Design review of the part built by this model. Coordinates are the model's own, in mm. Face numbers are marked on the shaded views. A direction names the side the tool comes from. Round coordinates to 2 decimals unless told otherwise and drop trailing zeros. Write each loop counter-clockwise with the first axis right and the second up, starting at its lowest first coordinate (ties: lowest second). Pieces come first, ordered by that corner, then holes. Notation, with made-up numbers: (64, 0) -> (98, 0) arc R27 cw to (98, 33) -> close; hole circle Ø7 at (-10, 29.5). An arc over 180 degrees is marked (long way). Write item = value, one per line. Start each with the question number.
Item 1: To check wall thickness, follow L1, parallel to Z at x = -17, y = 37; L2, parallel to X at y = -9.5, z = 28; L3, parallel to Y at x = -3.5, z = 21. State the ranges of each line that lie inside material, in increasing order.
Item 2: Add section D-D, the plane y = -2. State the section outline as (x, z) points.
Item 3: Mouldability with a two-part tool opening along Z and no side actions: class the marked faces 3, 4 and 5 as released by +Z, released by -Z, zero draft, split by the parting line, or undercut.
Item 4: For pin 1 Ø3 at (x, y) = (18, -42.5) entering from -Z; pin 2 Ø5 at (x, z) = (-5.5, 9.5) entering from -Y; pin 3 Ø12 at (x, y) = (-1, -25) entering from -Z; pin 4 Ø1.5 at (x, z) = (6.5, 17) entering from +Y, all flat-tipped, find the tip position at first contact; note any pin that passes through.
Item 5: Machinability: for the marked faces 1 and 2, which of the approach directions +Z, -Z, +X, -X, +Y, -Y give a long, thin tool a straight path to every point of the face, cutting with its end or side? Answer none if there is none.
Item 6: Add section A-A, the plane z = 9. State the section outline as (x, y) points.
Item 7: Add section C-C, the plane z = 17. State the section outline as (x, y) points.
Item 8: Add section B-B, the plane y = 36.5. State the section outline as (x, z) points, then the cut area to 3 significant figures.
from build123d import *

# Parameters (mm, degrees)
F0_W           = 41
F0_H           = 90
F1_DEPTH       = 34
F2_W           = 35
F2_H           = 29
F3_DEPTH       = 86
F4_W           = 7
F4_H           = 6
F4_R           = 1.55
F4_R_2         = 4
F5_DEPTH       = 4
F6_W           = 5
F6_H           = 2.5
F6_W_2         = 3
F6_H_2         = 5
F7_DEPTH       = 2.5
F8_W           = 5
F8_H           = 27
F9_DEPTH       = 4
F10_T4_DEPTH   = 29
F10_T10_DEPTH  = 29
F10_T16_DEPTH  = 29
F10_T23_DEPTH  = 29
F10_T29_DEPTH  = 29
F10_T35_DEPTH  = 29
F10_T41_DEPTH  = 29
F10_T47_DEPTH  = 29
F10_T54_DEPTH  = 29
F10_T60_DEPTH  = 29
F10_T66_DEPTH  = 35
F10_T72_DEPTH  = 35
F10_T78_DEPTH  = 35
F10_T85_DEPTH  = 35
F10_T91_DEPTH  = 35
F10_T97_DEPTH  = 35
F10_T103_DEPTH = 35
F10_T109_DEPTH = 35
F10_T116_DEPTH = 35
F10_T122_DEPTH = 35


# Not quite as in the source:
# - a fillet or chamfer that OpenCascade refuses, or shapes differently, is made with other operations: its cross-section is extruded or revolved along the edge and cut away or added


with BuildPart() as f1:
    # F0 (on Top) → F1 (new body)
    with BuildSketch(Plane.XY):
        with Locations((-1.7023412511, 4.193077401)):
            Rectangle(F0_W, F0_H)
    extrude(amount=F1_DEPTH)

    # F2 (on face) → F3 (cut)
    with BuildSketch(Plane.XZ.offset(40.806922599)):
        with Locations((-1.7023412511, 17)):
            Rectangle(F2_W, F2_H)
    extrude(amount=-F3_DEPTH, mode=Mode.SUBTRACT)

    # F4 (on face) → F5 (cut, through all)
    with BuildSketch(Plane(origin=(0, 49.193077401, 0), x_dir=(-1, 0, 0), z_dir=(0, 1, 0))):
        with Locations((-11.2976587489, 7)):
            Rectangle(F4_W, F4_H)
        with Locations((-7.7976587489, 17)):
            Circle(F4_R)
        with Locations((1.7023412511, 25)):
            Circle(F4_R)
        with Locations((1.7023412511, 17)):
            Circle(F4_R_2)
        with Locations((1.7023412511, 9)):
            Circle(F4_R)
        with Locations((11.2023412511, 17)):
            Circle(F4_R)
        with Locations((14.7023412511, 27)):
            Rectangle(F4_W, F4_H)
    extrude(amount=-F5_DEPTH, mode=Mode.SUBTRACT)

    # F6 (on face) → F7 (join)
    with BuildSketch(Plane.XZ.offset(40.806922599)):
        with Locations((-1.7023412511, 32.75)):
            Rectangle(F6_W, F6_H)
        with Locations((-20.7023412511, 17)):
            Rectangle(F6_W_2, F6_H_2)
        with Locations((17.2976587489, 17)):
            Rectangle(F6_W_2, F6_H_2)
        with Locations((-1.7023412511, 1.25)):
            Rectangle(F6_W, F6_H)
    extrude(amount=F7_DEPTH)

    # F8 (on face) → F9 (join)
    with BuildSketch(Plane(origin=(0, 0, 0), x_dir=(1, 0, 0), z_dir=(0, 0, -1))):
        with Locations((-19.7023412511, -9.693077401)):
            Rectangle(F8_W, F8_H)
        with Locations((16.2976587489, -9.693077401)):
            Rectangle(F8_W, F8_H)
    extrude(amount=F9_DEPTH)

    # F10: chamfer of 3 on 4 edges, made by hand


with BuildPart() as f10_tool2:
    # F10_s3 → F10_t4 (new body)
    with BuildSketch(Plane.XY.offset(31.5)):
        Polygon((-16.2023412511, 45.193077401), (-19.2023412511, 42.193077401), (-19.2023412511, 45.193077401), align=None)
    extrude(amount=-F10_T4_DEPTH)

    split(bisect_by=Plane.YZ.offset(-18.2023412511), keep=Keep.TOP)

    split(bisect_by=Plane.XY.offset(30), keep=Keep.TOP)


with BuildPart() as f1_1:
    add(f1.part)

    # F10_t1: union F10_tool2
    add(f10_tool2.part)


with BuildPart() as f10_tool8:
    # F10_s9 → F10_t10 (new body)
    with BuildSketch(Plane.XY.offset(31.5)):
        Polygon((-16.2023412511, 45.193077401), (-19.2023412511, 42.193077401), (-19.2023412511, 45.193077401), align=None)
    extrude(amount=-F10_T10_DEPTH)

    split(bisect_by=Plane.YZ.offset(-18.2023412511), keep=Keep.BOTTOM)

    split(bisect_by=Plane.XY.offset(30), keep=Keep.TOP)


with BuildPart() as f1_2:
    add(f1_1.part)

    # F10_t7: union F10_tool8
    add(f10_tool8.part)


with BuildPart() as f10_tool14:
    # F10_s15 → F10_t16 (new body)
    with BuildSketch(Plane.XY.offset(31.5)):
        Polygon((-16.2023412511, 45.193077401), (-19.2023412511, 42.193077401), (-19.2023412511, 45.193077401), align=None)
    extrude(amount=-F10_T16_DEPTH)

    split(bisect_by=Plane.YZ.offset(-18.2023412511), keep=Keep.BOTTOM)

    split(bisect_by=Plane.XY.offset(24), keep=Keep.TOP)

    split(bisect_by=Plane.XY.offset(30), keep=Keep.BOTTOM)


with BuildPart() as f1_3:
    add(f1_2.part)

    # F10_t13: union F10_tool14
    add(f10_tool14.part)


with BuildPart() as f10_tool21:
    # F10_s22 → F10_t23 (new body)
    with BuildSketch(Plane.XY.offset(31.5)):
        Polygon((-16.2023412511, 45.193077401), (-19.2023412511, 42.193077401), (-19.2023412511, 45.193077401), align=None)
    extrude(amount=-F10_T23_DEPTH)

    split(bisect_by=Plane.YZ.offset(-18.2023412511), keep=Keep.TOP)

    split(bisect_by=Plane.XY.offset(24), keep=Keep.BOTTOM)


with BuildPart() as f1_4:
    add(f1_3.part)

    # F10_t20: union F10_tool21
    add(f10_tool21.part)


with BuildPart() as f10_tool27:
    # F10_s28 → F10_t29 (new body)
    with BuildSketch(Plane.XY.offset(31.5)):
        Polygon((-16.2023412511, 45.193077401), (-19.2023412511, 42.193077401), (-19.2023412511, 45.193077401), align=None)
    extrude(amount=-F10_T29_DEPTH)

    split(bisect_by=Plane.YZ.offset(-18.2023412511), keep=Keep.BOTTOM)

    split(bisect_by=Plane.XY.offset(24), keep=Keep.BOTTOM)


with BuildPart() as f1_5:
    add(f1_4.part)

    # F10_t26: union F10_tool27
    add(f10_tool27.part)


with BuildPart() as f10_tool33:
    # F10_s34 → F10_t35 (new body)
    with BuildSketch(Plane.XY.offset(2.5)):
        Polygon((12.7976587489, 45.193077401), (15.7976587489, 42.193077401), (15.7976587489, 45.193077401), align=None)
    extrude(amount=F10_T35_DEPTH)

    split(bisect_by=Plane.XY.offset(4), keep=Keep.BOTTOM)

    split(bisect_by=Plane.YZ.offset(14.7976587489), keep=Keep.BOTTOM)


with BuildPart() as f1_6:
    add(f1_5.part)

    # F10_t32: union F10_tool33
    add(f10_tool33.part)


with BuildPart() as f10_tool39:
    # F10_s40 → F10_t41 (new body)
    with BuildSketch(Plane.XY.offset(2.5)):
        Polygon((12.7976587489, 45.193077401), (15.7976587489, 42.193077401), (15.7976587489, 45.193077401), align=None)
    extrude(amount=F10_T41_DEPTH)

    split(bisect_by=Plane.XY.offset(4), keep=Keep.BOTTOM)

    split(bisect_by=Plane.YZ.offset(14.7976587489), keep=Keep.TOP)


with BuildPart() as f1_7:
    add(f1_6.part)

    # F10_t38: union F10_tool39
    add(f10_tool39.part)


with BuildPart() as f10_tool45:
    # F10_s46 → F10_t47 (new body)
    with BuildSketch(Plane.XY.offset(2.5)):
        Polygon((12.7976587489, 45.193077401), (15.7976587489, 42.193077401), (15.7976587489, 45.193077401), align=None)
    extrude(amount=F10_T47_DEPTH)

    split(bisect_by=Plane.XY.offset(4), keep=Keep.TOP)

    split(bisect_by=Plane.YZ.offset(14.7976587489), keep=Keep.TOP)

    split(bisect_by=Plane.XY.offset(10), keep=Keep.BOTTOM)


with BuildPart() as f1_8:
    add(f1_7.part)

    # F10_t44: union F10_tool45
    add(f10_tool45.part)


with BuildPart() as f10_tool52:
    # F10_s53 → F10_t54 (new body)
    with BuildSketch(Plane.XY.offset(2.5)):
        Polygon((12.7976587489, 45.193077401), (15.7976587489, 42.193077401), (15.7976587489, 45.193077401), align=None)
    extrude(amount=F10_T54_DEPTH)

    split(bisect_by=Plane.YZ.offset(14.7976587489), keep=Keep.BOTTOM)

    split(bisect_by=Plane.XY.offset(10), keep=Keep.TOP)


with BuildPart() as f1_9:
    add(f1_8.part)

    # F10_t51: union F10_tool52
    add(f10_tool52.part)


with BuildPart() as f10_tool58:
    # F10_s59 → F10_t60 (new body)
    with BuildSketch(Plane.XY.offset(2.5)):
        Polygon((12.7976587489, 45.193077401), (15.7976587489, 42.193077401), (15.7976587489, 45.193077401), align=None)
    extrude(amount=F10_T60_DEPTH)

    split(bisect_by=Plane.YZ.offset(14.7976587489), keep=Keep.TOP)

    split(bisect_by=Plane.XY.offset(10), keep=Keep.TOP)


with BuildPart() as f1_10:
    add(f1_9.part)

    # F10_t57: union F10_tool58
    add(f10_tool58.part)


with BuildPart() as f10_tool64:
    # F10_s65 → F10_t66 (new body)
    with BuildSketch(Plane.YZ.offset(15.7976587489)):
        Polygon((45.193077401, 28.5), (42.193077401, 31.5), (45.193077401, 31.5), align=None)
    extrude(amount=-F10_T66_DEPTH)

    split(bisect_by=Plane.YZ.offset(-11.2023412511), keep=Keep.TOP)

    split(bisect_by=Plane.XY.offset(30), keep=Keep.BOTTOM)


with BuildPart() as f1_11:
    add(f1_10.part)

    # F10_t63: union F10_tool64
    add(f10_tool64.part)


with BuildPart() as f10_tool70:
    # F10_s71 → F10_t72 (new body)
    with BuildSketch(Plane.YZ.offset(15.7976587489)):
        Polygon((45.193077401, 28.5), (42.193077401, 31.5), (45.193077401, 31.5), align=None)
    extrude(amount=-F10_T72_DEPTH)

    split(bisect_by=Plane.YZ.offset(-11.2023412511), keep=Keep.TOP)

    split(bisect_by=Plane.XY.offset(30), keep=Keep.TOP)


with BuildPart() as f1_12:
    add(f1_11.part)

    # F10_t69: union F10_tool70
    add(f10_tool70.part)


with BuildPart() as f10_tool76:
    # F10_s77 → F10_t78 (new body)
    with BuildSketch(Plane.YZ.offset(15.7976587489)):
        Polygon((45.193077401, 28.5), (42.193077401, 31.5), (45.193077401, 31.5), align=None)
    extrude(amount=-F10_T78_DEPTH)

    split(bisect_by=Plane.YZ.offset(-18.2023412511), keep=Keep.TOP)

    split(bisect_by=Plane.YZ.offset(-11.2023412511), keep=Keep.BOTTOM)

    split(bisect_by=Plane.XY.offset(30), keep=Keep.TOP)


with BuildPart() as f1_13:
    add(f1_12.part)

    # F10_t75: union F10_tool76
    add(f10_tool76.part)


with BuildPart() as f10_tool83:
    # F10_s84 → F10_t85 (new body)
    with BuildSketch(Plane.YZ.offset(15.7976587489)):
        Polygon((45.193077401, 28.5), (42.193077401, 31.5), (45.193077401, 31.5), align=None)
    extrude(amount=-F10_T85_DEPTH)

    split(bisect_by=Plane.YZ.offset(-18.2023412511), keep=Keep.BOTTOM)

    split(bisect_by=Plane.XY.offset(30), keep=Keep.BOTTOM)


with BuildPart() as f1_14:
    add(f1_13.part)

    # F10_t82: union F10_tool83
    add(f10_tool83.part)


with BuildPart() as f10_tool89:
    # F10_s90 → F10_t91 (new body)
    with BuildSketch(Plane.YZ.offset(15.7976587489)):
        Polygon((45.193077401, 28.5), (42.193077401, 31.5), (45.193077401, 31.5), align=None)
    extrude(amount=-F10_T91_DEPTH)

    split(bisect_by=Plane.YZ.offset(-18.2023412511), keep=Keep.BOTTOM)

    split(bisect_by=Plane.XY.offset(30), keep=Keep.TOP)


with BuildPart() as f1_15:
    add(f1_14.part)

    # F10_t88: union F10_tool89
    add(f10_tool89.part)


with BuildPart() as f10_tool95:
    # F10_s96 → F10_t97 (new body)
    with BuildSketch(Plane.YZ.offset(-19.2023412511)):
        Polygon((45.193077401, 5.5), (42.193077401, 2.5), (45.193077401, 2.5), align=None)
    extrude(amount=F10_T97_DEPTH)

    split(bisect_by=Plane.YZ.offset(7.7976587489), keep=Keep.BOTTOM)

    split(bisect_by=Plane.XY.offset(4), keep=Keep.TOP)


with BuildPart() as f1_16:
    add(f1_15.part)

    # F10_t94: union F10_tool95
    add(f10_tool95.part)


with BuildPart() as f10_tool101:
    # F10_s102 → F10_t103 (new body)
    with BuildSketch(Plane.YZ.offset(-19.2023412511)):
        Polygon((45.193077401, 5.5), (42.193077401, 2.5), (45.193077401, 2.5), align=None)
    extrude(amount=F10_T103_DEPTH)

    split(bisect_by=Plane.YZ.offset(7.7976587489), keep=Keep.BOTTOM)

    split(bisect_by=Plane.XY.offset(4), keep=Keep.BOTTOM)


with BuildPart() as f1_17:
    add(f1_16.part)

    # F10_t100: union F10_tool101
    add(f10_tool101.part)


with BuildPart() as f10_tool107:
    # F10_s108 → F10_t109 (new body)
    with BuildSketch(Plane.YZ.offset(-19.2023412511)):
        Polygon((45.193077401, 5.5), (42.193077401, 2.5), (45.193077401, 2.5), align=None)
    extrude(amount=F10_T109_DEPTH)

    split(bisect_by=Plane.YZ.offset(7.7976587489), keep=Keep.TOP)

    split(bisect_by=Plane.XY.offset(4), keep=Keep.BOTTOM)

    split(bisect_by=Plane.YZ.offset(14.7976587489), keep=Keep.BOTTOM)


with BuildPart() as f1_18:
    add(f1_17.part)

    # F10_t106: union F10_tool107
    add(f10_tool107.part)


with BuildPart() as f10_tool114:
    # F10_s115 → F10_t116 (new body)
    with BuildSketch(Plane.YZ.offset(-19.2023412511)):
        Polygon((45.193077401, 5.5), (42.193077401, 2.5), (45.193077401, 2.5), align=None)
    extrude(amount=F10_T116_DEPTH)

    split(bisect_by=Plane.XY.offset(4), keep=Keep.TOP)

    split(bisect_by=Plane.YZ.offset(14.7976587489), keep=Keep.TOP)


with BuildPart() as f1_19:
    add(f1_18.part)

    # F10_t113: union F10_tool114
    add(f10_tool114.part)


with BuildPart() as f10_tool120:
    # F10_s121 → F10_t122 (new body)
    with BuildSketch(Plane.YZ.offset(-19.2023412511)):
        Polygon((45.193077401, 5.5), (42.193077401, 2.5), (45.193077401, 2.5), align=None)
    extrude(amount=F10_T122_DEPTH)

    split(bisect_by=Plane.XY.offset(4), keep=Keep.BOTTOM)

    split(bisect_by=Plane.YZ.offset(14.7976587489), keep=Keep.TOP)


with BuildPart() as f1_20:
    add(f1_19.part)

    # F10_t119: union F10_tool120
    add(f10_tool120.part)


solid = f1_20.part
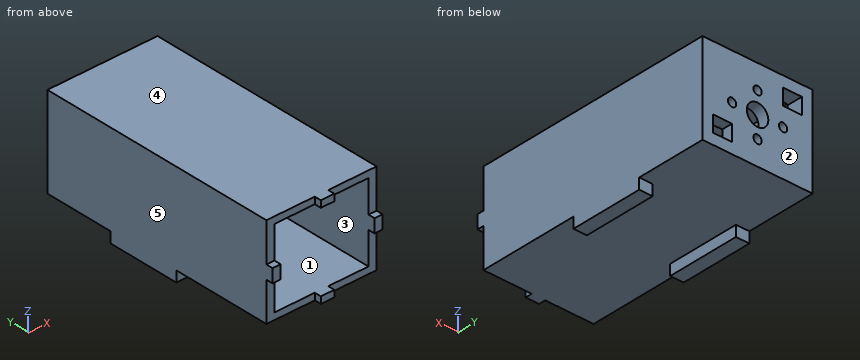
Result set:
q1.L1 = 0 to 2.5, 31.5 to 34
q1.L2 = -22.2 to -19.2, 15.8 to 18.8
q1.L3 = 45.19 to 49.19
q2.outline = (-22.2, -4) -> (-17.2, -4) -> (-17.2, 0) -> (13.8, 0) -> (13.8, -4) -> (18.8, -4) -> (18.8, 34) -> (-22.2, 34) -> close; hole (-19.2, 2.5) -> (15.8, 2.5) -> (15.8, 31.5) -> (-19.2, 31.5) -> close
q3.face_3 = undercut
q3.face_4 = released by +Z
q3.face_5 = zero draft
q4.pin_1 = 14.5
q4.pin_2 = 45.19
q4.pin_3 = 0
q4.pin_4 = 49.19
q5.face_1 = -Y
q5.face_2 = +Z, -Z, +X, -X, +Y
q6.outline = (-22.2, -40.81) -> (-19.2, -40.81) -> (-19.2, 42.19) -> (-16.2, 45.19) -> (-3.25, 45.19) -> (-3.25, 49.19) -> (-22.2, 49.19) -> close; (-0.15, 45.19) -> (7.8, 45.19) -> (7.8, 49.19) -> (-0.15, 49.19) -> close; (14.8, 43.19) -> (15.8, 42.19) -> (15.8, -40.81) -> (18.8, -40.81) -> (18.8, 49.19) -> (14.8, 49.19) -> close
q7.outline = (-22.2, -43.31) -> (-19.2, -43.31) -> (-19.2, 42.19) -> (-16.2, 45.19) -> (-12.75, 45.19) -> (-12.75, 49.19) -> (-22.2, 49.19) -> close; (-9.65, 45.19) -> (-5.7, 45.19) -> (-5.7, 49.19) -> (-9.65, 49.19) -> close; (2.3, 45.19) -> (6.25, 45.19) -> (6.25, 49.19) -> (2.3, 49.19) -> close; (9.35, 45.19) -> (12.8, 45.19) -> (15.8, 42.19) -> (15.8, -43.31) -> (18.8, -43.31) -> (18.8, 49.19) -> (9.35, 49.19) -> close
q8.outline = (-22.2, 0) -> (18.8, 0) -> (18.8, 34) -> (-22.2, 34) -> close; hole (-19.2, 2.5) -> (15.8, 2.5) -> (15.8, 31.5) -> (-19.2, 31.5) -> close
q8.area = 379 mm²
